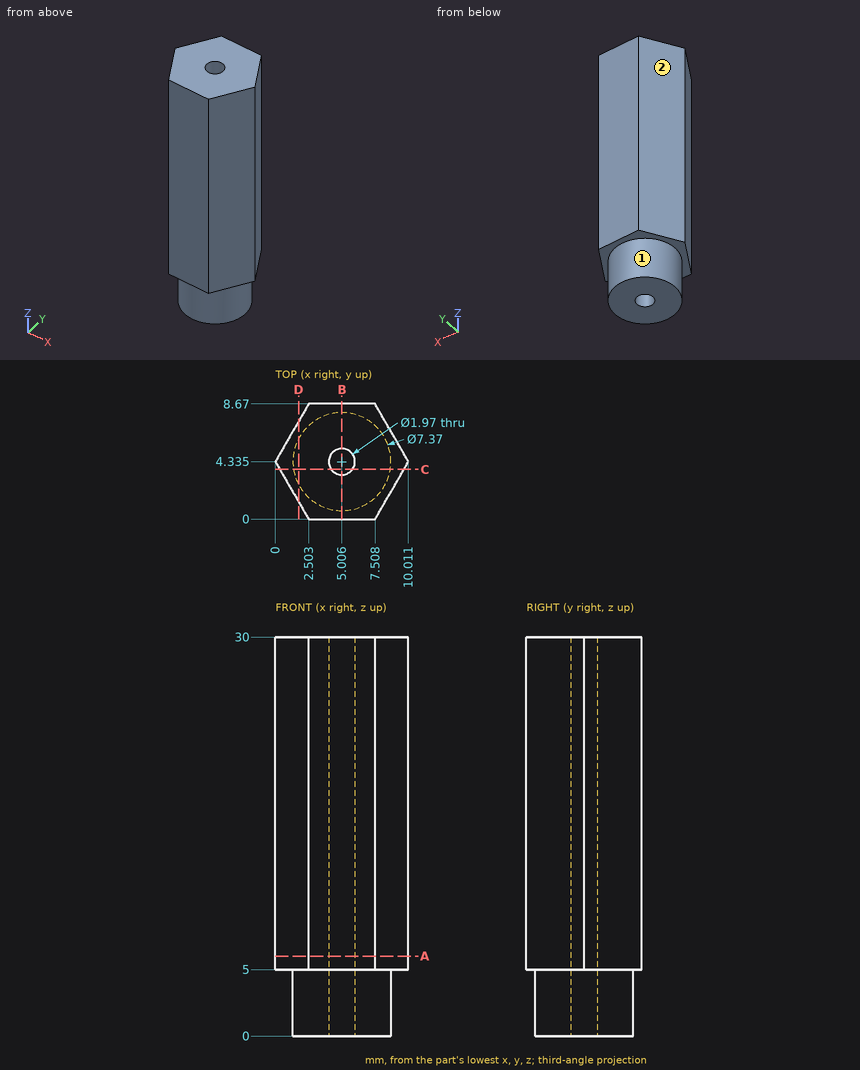
The figure shows three views and two pictorial views of one solid part (mm, origin at its lowest corner). Answer the questions. A direction names the side the tool comes from. Round coordinates to 2 decimals unless told otherwise and drop trailing zeros. Write each loop counter-clockwise with the first axis right and the second up, starting at its lowest first coordinate (ties: lowest second). Pieces come first, ordered by that corner, then holes. Notation, with made-up numbers: M 13,23.5 L 65,23.5 A20 ccw 65,30.5 Z; hole C 72,62 d1. An arc over 180 degrees is marked long. Write each question's results on one line, items separated by ' | '. Start each with the question number.
(1) The part is cut by section B-B, the plane x = 5. Write down the section's boundary in (y, z).
(2) The part is cut by section D-D, the plane x = 1.75. Write down the section's boundary in (y, z).
(3) This flat-tipped pin is pushed along its axis until it touches: P1, Ø3, axis at y = 7.5, z = 21.5, coming from the -X side. Where does it stop, or does it pass through?
(4) Find the intervals of material crossed by line 1 (Y direction, x = 5, z = 9.25); line 2 (Z direction, x = 9.25, y = 4.5); line 3 (X direction, y = 4.5, z = 28) (1 decimal), in increasing order.
(5) For the marked faces 1 and 2, determine the directions among +Z, -Z, +X, -X, +Y, -Y from which every point of the face is accessible in a straight line to the end or side of a thin tool.
(6) The part is cut by section A-A, the plane z = 6. Write down the section's boundary in (x, y) (1 decimal).
(7) The part is cut by section C-C, the plane y = 3.75. Write down the section's boundary in (x, z).
Worked answers:
1) outline: M 0,5 L 0.65,5 L 0.65,0 L 3.35,0 L 3.35,30 L 0,30 Z; M 5.32,0 L 8.02,0 L 8.02,5 L 8.67,5 L 8.67,30 L 5.32,30 Z
2) outline: M 1.3,5 L 2.61,5 L 2.61,0 L 6.06,0 L 6.06,5 L 7.37,5 L 7.37,30 L 1.3,30 Z
3) P1: stops at x = 0.96
4) line 1: y = 0 to 3.35, 5.32 to 8.67 | line 2: z = 5 to 30 | line 3: x = 0.1 to 4, 6 to 9.9
5) face 1: -Z | face 2: +Z, -Z, -X, +Y
6) outline: M 0,4.3 L 2.5,0 L 7.5,0 L 10,4.3 L 7.5,8.7 L 2.5,8.7 Z; hole C 5,4.3 d2
7) outline: M 0.34,5 L 1.37,5 L 1.37,0 L 4.21,0 L 4.21,30 L 0.34,30 Z; M 5.8,0 L 8.64,0 L 8.64,5 L 9.67,5 L 9.67,30 L 5.8,30 Z
